```python
from build123d import *

# Parameters (mm, degrees)
SKETCH003_R        = 1.5
PAD001_DEPTH       = 10
SKETCH_R           = 5.004015
PAD_DEPTH          = 12
SKETCH001_W        = 11.284618
SKETCH001_H        = 1.110598
POCKET_DEPTH       = 5
POLARPATTERN_COUNT = 2
POLARPATTERN_ANGLE = 90
SKETCH002_R        = 3
POCKET001_DEPTH    = 5


with BuildPart() as revolution:
    # Sketch004 → Revolution (revolve)
    with BuildSketch(Plane.XZ):
        with BuildLine():
            ThreePointArc((0, -0.399672), (3.65233, 1.175436), (5.120847, 4.871912))
            Line((5.120847, 4.871912), (6.070016, 4.871912))
            Line((6.070016, 4.871912), (6.070016, -2.113572))
            Line((0, -2.113572), (6.070016, -2.113572))
            Line((0, -0.399672), (0, -2.113572))
        make_face()
    revolve(axis=Axis((0, 0, 0), (0, 0, 1)))


with BuildPart() as pad001:
    # Sketch003 → Pad001 (new body, symmetric)
    with BuildSketch(Plane.XZ):
        with Locations((0, 2.5)):
            Circle(SKETCH003_R)
    extrude(amount=PAD001_DEPTH, both=True)


with BuildPart() as obj1:
    # Sketch → Pad (new body)
    with BuildSketch(Plane.XY):
        Circle(SKETCH_R)
    extrude(amount=PAD_DEPTH)

    # Sketch001 → Pocket (cut)
    with BuildSketch(Plane.XY.offset(12)):
        Rectangle(SKETCH001_W, SKETCH001_H)
    pocket = extrude(amount=-POCKET_DEPTH, mode=Mode.SUBTRACT)

    # PolarPattern: Pocket ×2 about axis
    polarpattern_axis = Axis((0, 0, 12), (0, 0, 1))
    for i in range(1, POLARPATTERN_COUNT):
        add(pocket.rotate(polarpattern_axis, i * POLARPATTERN_ANGLE / (POLARPATTERN_COUNT - 1)), mode=Mode.SUBTRACT)

    # Sketch002 → Pocket001 (cut)
    with BuildSketch(Plane.XY.offset(12)):
        with Locations((0.003381, 0.006761)):
            Circle(SKETCH002_R)
    extrude(amount=-POCKET001_DEPTH, mode=Mode.SUBTRACT)

    # Cut: cut Pad001
    add(pad001.part, mode=Mode.SUBTRACT)

    # Cut001: cut Revolution
    add(revolution.part, mode=Mode.SUBTRACT)


solid = obj1.part
```
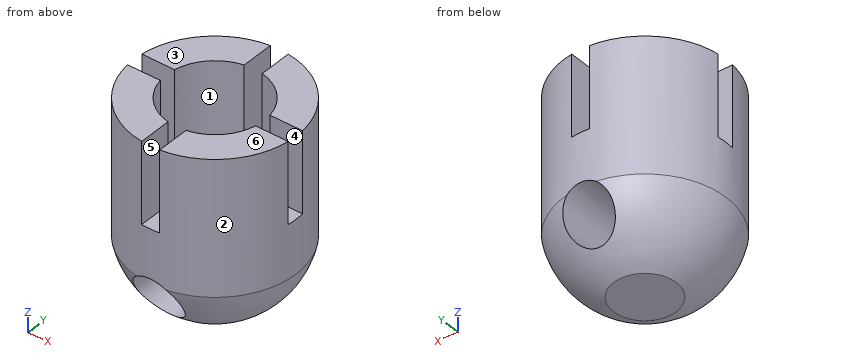
Source: CAD feature listing. Evaluate the final solid. Frame: model axes, mm. Face numbers are marked on the shaded views. A direction names the side the tool comes from. Round coordinates to 2 decimals unless told otherwise and drop trailing zeros. Loops run counter-clockwise (first coordinate to the right, second up) from the corner with the lowest first, then second, coordinate; pieces in that order, holes last. Notation, with made-up numbers: M 74.25,44 L 110.25,44 A34 cw 110.25,79 Z; hole C 59,40 d6. An arc over 180 degrees is marked long. Put each result on its own line as item: value.
(1) First-contact query: pin 1 (2 mm diameter, centred on y = 3.5, z = 7, fed in from -X); pin 2 (1 mm diameter, centred on x = -0.5, y = -4, fed in from -Z); pin 3 (0.6 mm diameter, centred on x = -4, z = 9, fed in from -Y); pin 4 (1.8 mm diameter, centred on x = 0, z = 2.5, fed in from -Y). Flat tips, straight axial feed; report the tip coordinate or a pass-through.
Solutions:
pin 1: x = -4.33
pin 2: z = 1.05
pin 3: y = -3.37
pin 4: through
(2) Section A-A, the plane z = 9.25. Return loops of the section in (x, y).
Solutions:
outline: M -4.97,-0.56 A5 ccw -0.56,-4.97 L -0.56,-2.94 A3 cw -2.94,-0.56 Z; M -4.97,0.56 L -2.95,0.56 A3 cw -0.56,2.95 L -0.56,4.97 A5 ccw Z; M 0.56,-4.97 A5 ccw 4.97,-0.56 L 2.95,-0.56 A3 cw 0.56,-2.94 Z; M 0.56,2.96 A3 cw 2.95,0.56 L 4.97,0.56 A5 ccw 0.56,4.97 Z
(3) Section B-B, the plane z = 6. Return loops of the section in (x, y).
Solutions:
outline: C 0,0 d10.01
(4) Access query for the marked faces 4, 5 and 6. Directions: +Z, -Z, +X, -X, +Y, -Y. A direction counts if a zero-diameter tool reaches every point of the face in a straight line with its end or side. Return the directions, or none.
Solutions:
face 4: +Z, +X, -X
face 5: +Z, +Y, -Y
face 6: +Z, +X, -X, +Y, -Y
(5) Pull-direction query (Y, two-part tool) for the marked faces 1, 2 and 3; classes: released by +Y, released by -Y, zero draft, split by the parting line, or undercut.
Solutions:
face 1: undercut
face 2: split by the parting line
face 3: zero draft
(6) Ray query, line 1 (Z direction, x = 0, y = -1.25); line 2 (Y direction, x = -3.25, z = 10.5); line 3 (X direction, y = 2.25, z = 3.5). Return the intervals inside material, ascending. Write a range as [from, to].
Solutions:
line 1: [0, 1], [4, 7]
line 2: [-3.8, -0.56], [0.56, 3.8]
line 3: [-4.42, -1.12], [1.12, 4.42]
